Geometry check sheet. Reference: drawing and pictorial views, mm from the part's lowest x, y, z. A direction names the side the tool comes from. Give positions to 0.01 mm unless a question says otherwise; leave off trailing zeros. Write each loop counter-clockwise with the first axis right and the second up, starting at its lowest first coordinate (ties: lowest second). Pieces come first, ordered by that corner, then holes. Notation, with made-up numbers: (60.5, 37) - (117.5, 37) arc R16 cw to (117.5, 63) - close; hole circle Ø2 at (-27.5, 22). An arc over 180 degrees is marked (long way). Put each result on its own line as item: value.
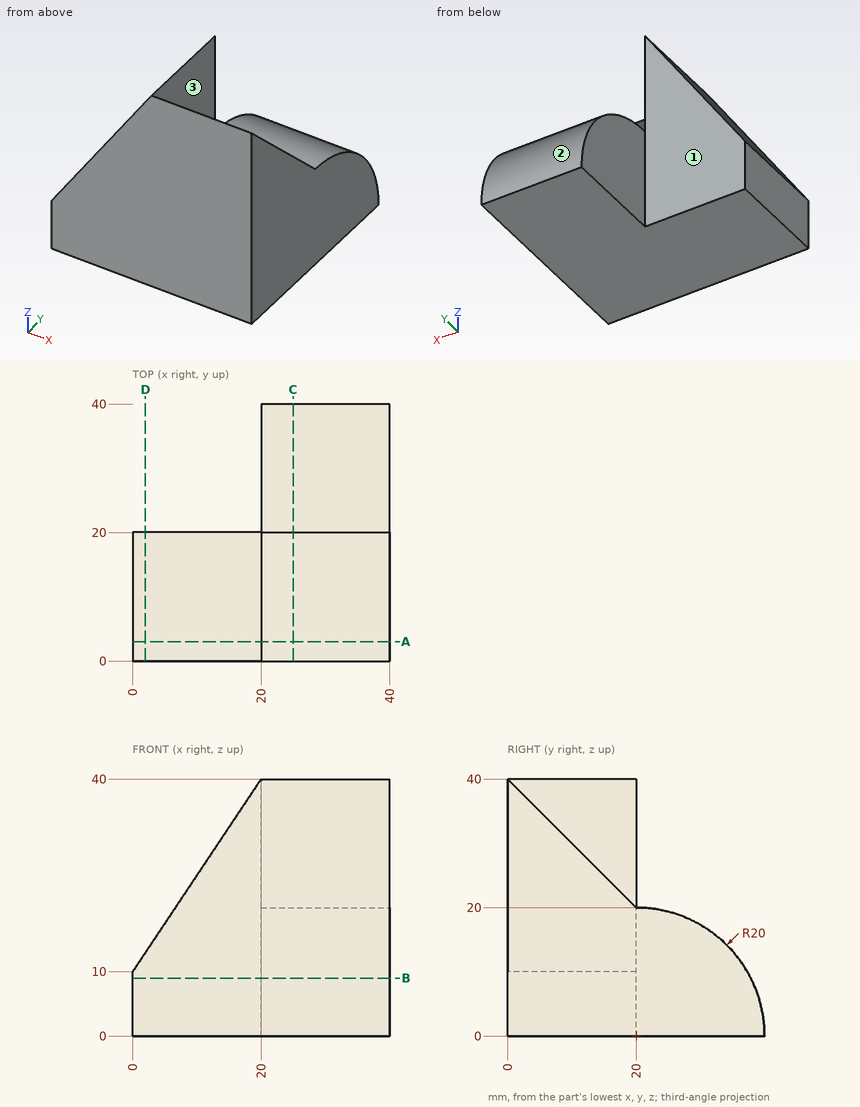
Q1. Section check D-D, the plane x = 2. Record the cut outline in (y, z), plus the area to 3 significant figures.
Answers follow:
outline: (0, 0) - (20, 0) - (20, 13) - (0, 13) - close
area: 260 mm2
Q2. Go/stop test with flat-tipped pins: pin 1 Ø22 at (x, z) = (6, 20.5) entering from +Y; pin 2 Ø1 at (x, z) = (33, 21) entering from +Y; pin 3 Ø3 at (x, y) = (24, 31.5) entering from +Z. Record where each tip stops, or that it passes through.
Answers follow:
pin 1: stops at y = 20
pin 2: stops at y = 19.5
pin 3: stops at z = 17.32
Q3. Set-up check for the marked faces 1, 2 and 3: record each of +Z, -Z, +X, -X, +Y, -Y from which the full face is reachable in a straight line by a thin tool's end or side.
Answers follow:
face 1: +Z, -Z, -X, +Y
face 2: +Z, +X, -X, +Y
face 3: +Z, +X, +Y
Q4. Scan lines: line 1 along X through (y, z) = (26.5, 13); line 2 along Y through (x, z) = (17, 15.5); line 3 along Y through (x, z) = (34.5, 24). Record each from-to range of solid material in increasing order.
Answers follow:
line 1: x = 20 to 40
line 2: y = 0 to 20
line 3: y = 0 to 16
Q5. Section check C-C, the plane x = 25. Record the cut outline in (y, z), plus the area to 3 significant figures.
Answers follow:
outline: (0, 0) - (40, 0) arc R20 ccw to (20, 20) - (0, 40) - close
area: 914 mm2
Q6. Section check B-B, the plane z = 9. Record the cut outline in (x, y).
Answers follow:
outline: (0, 0) - (40, 0) - (40, 37.86) - (20, 37.86) - (20, 20) - (0, 20) - close
Q7. Section check A-A, the plane y = 3. Record the cut outline in (x, z), plus the area to 3 significant figures.
Answers follow:
outline: (0, 0) - (40, 0) - (40, 37) - (20, 37) - (20, 40) - (0, 10) - close
area: 1,240 mm2
